```python
from build123d import *

# Parameters (mm, degrees)
SKETCH_1_W          = 120
SKETCH_1_H          = 120
EXTRUDE_1_DEPTH     = 3
SKETCH_2_R          = 2
SKETCH_2_R_2        = 6.5
SKETCH_2_R_3        = 2.6
SKETCH_2_W          = 51
SKETCH_2_H          = 57
CUT_EXTRUDE_1_DEPTH = 3


with BuildPart() as part:
    # 草图1 → 凸台-拉伸1 (new body)
    with BuildSketch(Plane(origin=(0, 0, 0), x_dir=(1, 0, 0), z_dir=(0, 1, 0))):
        with Locations((60, -60)):
            Rectangle(SKETCH_1_W, SKETCH_1_H)
    extrude(amount=EXTRUDE_1_DEPTH)

    # 草图2 → 切除-拉伸1 (cut)
    with BuildSketch(Plane(origin=(0, 3, 0), x_dir=(1, 0, 0), z_dir=(0, 1, 0))):
        with Locations((20, -88)):
            Circle(SKETCH_2_R)
        with Locations((95, -88)):
            Circle(SKETCH_2_R_2)
        with Locations((32.086613668, -8.5)):
            Circle(SKETCH_2_R_3)
        with Locations((32.086613668, -52.5)):
            Circle(SKETCH_2_R_3)
        with Locations((90.086613668, -8.5)):
            Circle(SKETCH_2_R_3)
        with Locations((90.086613668, -52.5)):
            Circle(SKETCH_2_R_3)
        with Locations((61.086613668, -28.5)):
            Rectangle(SKETCH_2_W, SKETCH_2_H)
    extrude(amount=-CUT_EXTRUDE_1_DEPTH, mode=Mode.SUBTRACT)


solid = part.part
```
Geometry: final body of the model. Coordinates: model frame, mm. A direction names the side the tool comes from. Round coordinates to 2 decimals unless told otherwise and drop trailing zeros. Write each loop counter-clockwise with the first axis right and the second up, starting at its lowest first coordinate (ties: lowest second). Pieces come first, ordered by that corner, then holes.
Item 1: Material intervals for L1, parallel to X at y = 1.55, z = 46.5; L2, parallel to X at y = 1.75, z = 88; L3, parallel to Z at x = 33, y = 1, sorted ascending.
Item 2: Section query B-B (y = 0.9). Return loops of the section in (x, z).
Item 3: Section query A-A (x = 95). Return loops of the section in (y, z).
Item 4: Pin query (flat end, axial travel): P1, Ø3, axis at x = 90.09, z = 8.5, coming from the -Y side; P2, Ø1.5, axis at x = 60, y = 2, coming from the -Z side. Return the tip coordinate at first contact, or that it passes through.
Item 5: Set-up query: faces 5 (the face through (86.587, 2, 29)), 6 (the face through (34.488, 1.521, 53.496)). Return all of +Z, -Z, +X, -X, +Y, -Y with unobstructed straight access to the full face (end or side cutting, diameter ignored); none if empty.
Item 6: Mould query, pull axis X, two halves, no side actions, for faces 1 (the face through (0, 1, 61)), 2 (the face through (59, 0, 72)), 3 (the face through (92.567, 1.521, 7.719)), 4 (the face through (120, 1, 61)). Classes: +X half, -X half, draft (parallel to the pull), parting line (faces both ways), or undercut.
Item 7: Section query D-D (z = 52.5). Return loops of the section in (x, y), plus the area to 3 significant figures.
Item 8: Section query C-C (z = 88). Return loops of the section in (x, y).
Completed:
1. L1: x = 0 to 35.59, 86.59 to 120
1. L2: x = 0 to 18, 22 to 88.5, 101.5 to 120
1. L3: z = 0 to 6.07, 10.93 to 50.07, 54.93 to 120
2. outline: (0, 0) - (35.59, 0) - (35.59, 57) - (86.59, 57) - (86.59, 0) - (120, 0) - (120, 120) - (0, 120) - close; hole circle Ø4 at (20, 88); hole circle Ø5.2 at (32.09, 8.5); hole circle Ø5.2 at (32.09, 52.5); hole circle Ø5.2 at (90.09, 8.5); hole circle Ø5.2 at (90.09, 52.5); hole circle Ø13 at (95, 88)
3. outline: (0, 0) - (3, 0) - (3, 81.5) - (0, 81.5) - close; (0, 94.5) - (3, 94.5) - (3, 120) - (0, 120) - close
4. P1: passes through
4. P2: stops at z = 57
5. face 5: -Z, +Y, -Y
5. face 6: +Y, -Y
6. face 1: -X half
6. face 2: draft
6. face 3: undercut
6. face 4: +X half
7. outline: (0, 0) - (29.49, 0) - (29.49, 3) - (0, 3) - close; (34.69, 0) - (35.59, 0) - (35.59, 3) - (34.69, 3) - close; (86.59, 0) - (87.49, 0) - (87.49, 3) - (86.59, 3) - close; (92.69, 0) - (120, 0) - (120, 3) - (92.69, 3) - close
7. area: 176 mm2
8. outline: (0, 0) - (18, 0) - (18, 3) - (0, 3) - close; (22, 0) - (88.5, 0) - (88.5, 3) - (22, 3) - close; (101.5, 0) - (120, 0) - (120, 3) - (101.5, 3) - close
